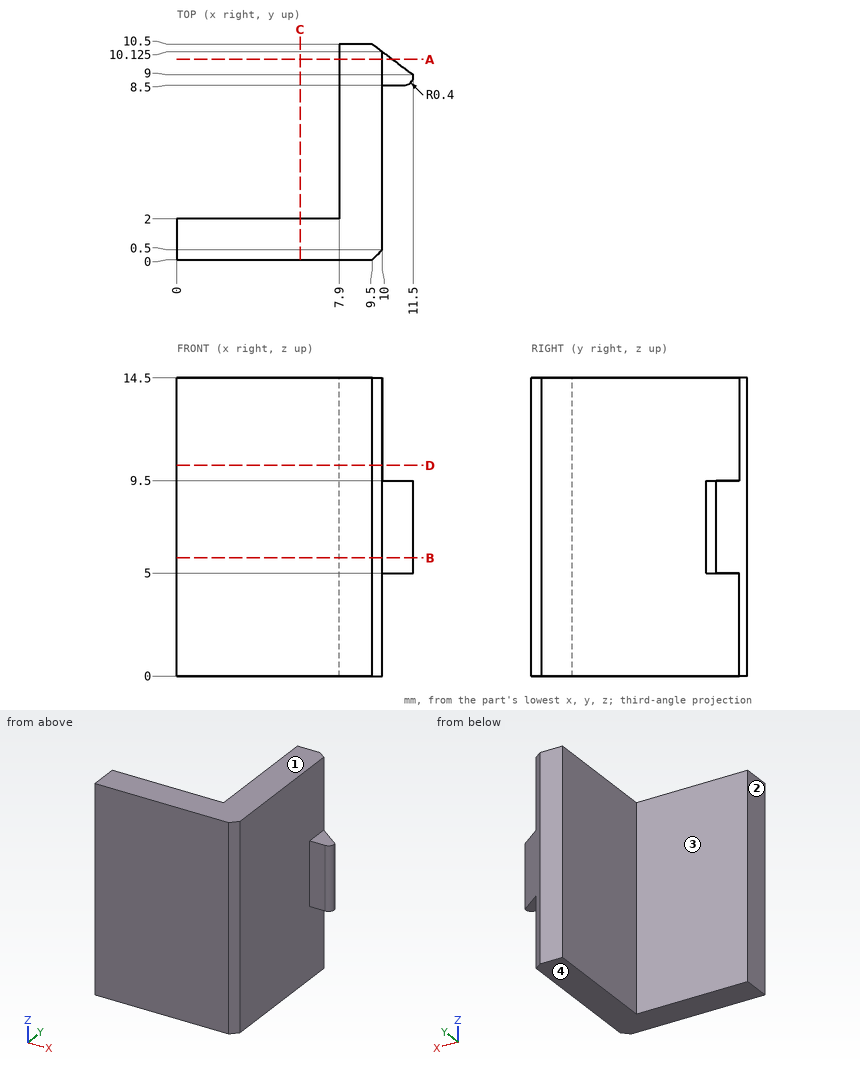
Job drawing, mm, ordinate dimensions from the low corner. One solid piece. A direction names the side the tool comes from. Round coordinates to 2 decimals unless told otherwise and drop trailing zeros. Order: outer loops, then holes, each group sorted by start corner. A loop starts at its lowest first (then second) coordinate and runs counter-clockwise, first axis right, second up. Notation, with made-up numbers: (75, 23) - (90, 23) arc R27 cw to (90, 55) - close; hole circle Ø2 at (25.5, 49.25). An arc over 180 degrees is marked (long way). Use CSV: the item, a comma, the result in double quotes. Start each with the question number.
1) Saw through at C-C (x = 6). List the corners of the cut face in (y, z).
2) Saw through at B-B (z = 5.75). List the corners of the cut face in (x, y).
3) Saw through at A-A (y = 9.75). List the corners of the cut face in (x, z).
4) Two-plate mould, pull along X, no slides. Class the marked faces 1 and 2: pulls with the +X half, pulls with the -X half, needs draft (parallel to the pull), parting line crosses it, or undercut.
5) Wall check: L1, parallel to X at y = 5, z = 13; L2, parallel to X at y = 1.5, z = 12.75; L3, parallel to Y at x = 5.25, z = 13. Give the ranges that are in metal, low to high. Write a range as [from, to].
6) Pin check, flat tips, straight feed: pin 1 Ø2 at (x, y) = (10.5, 7.5) entering from -Z; pin 2 Ø1.2 at (x, z) = (11, 7) entering from -Y; pin 3 Ø4 at (x, z) = (5.5, 9) entering from +Y; pin 4 Ø3 at (y, z) = (4, 9.5) entering from -X. Stop position of each tip, or through.
7) Saw through at D-D (z = 10.25). List the corners of the cut face in (x, y) (3 decimals).
8) Tool access for the marked faces 3 and 4: list every direction of +Z, -Z, +X, -X, +Y, -Y with a clear straight run to the whole face (end or side of a thin tool).
Values follow:
1,outline,"(0, 0) - (2, 0) - (2, 14.5) - (0, 14.5) - close"
2,outline,"(0, 0) - (9.5, 0) - (10, 0.5) - (10, 8.5) - (11.1, 8.5) arc R0.4 ccw to (11.5, 8.9) - (11.5, 9) - (9.5, 10.5) - (7.9, 10.5) - (7.9, 2) - (0, 2) - close"
3,outline,"(7.9, 0) - (10, 0) - (10, 5) - (10.5, 5) - (10.5, 9.5) - (10, 9.5) - (10, 14.5) - (7.9, 14.5) - close"
4,face 1,"needs draft"
4,face 2,"pulls with the -X half"
5,L1,"x = [7.9, 10]"
5,L2,"x = [0, 10]"
5,L3,"y = [0, 2]"
6,pin 1,"stops at z = 0"
6,pin 2,"stops at y = 8.5"
6,pin 3,"stops at y = 2"
6,pin 4,"stops at x = 7.9"
7,outline,"(0, 0) - (9.5, 0) - (10, 0.5) - (10, 10.125) - (9.5, 10.5) - (7.9, 10.5) - (7.9, 2) - (0, 2) - close"
8,face 3,"+Z, -Z, -X, +Y"
8,face 4,"-Z, +X, -X, +Y, -Y"
